from build123d import *

# Parameters (mm, degrees)
BOSS_EXTRUDE1_DEPTH = 3.5
BOSS_EXTRUDE2_DEPTH = 1.5
BOSS_EXTRUDE2_TAPER = 7


with BuildPart() as part:
    # Sketch1 → Boss-Extrude1 (new body)
    with BuildSketch(Plane.XY):
        Polygon((-2.95, 2), (-1.95, 3), (1.95, 3), (2.95, 2), (2.95, -2), (1.95, -3), (-1.95, -3), (-2.95, -2), align=None)
    extrude(amount=BOSS_EXTRUDE1_DEPTH)

    # Sketch2 → Boss-Extrude2 (add)
    with BuildSketch(Plane.XY.offset(3.5)):
        Polygon((-2.5, 1.7), (-2.5, -1.7), (-1.75, -2.45), (1.75, -2.45), (2.5, -1.7), (2.5, 1.7), (1.75, 2.45), (-1.75, 2.45), align=None)
    extrude(amount=BOSS_EXTRUDE2_DEPTH, taper=BOSS_EXTRUDE2_TAPER)


solid = part.part
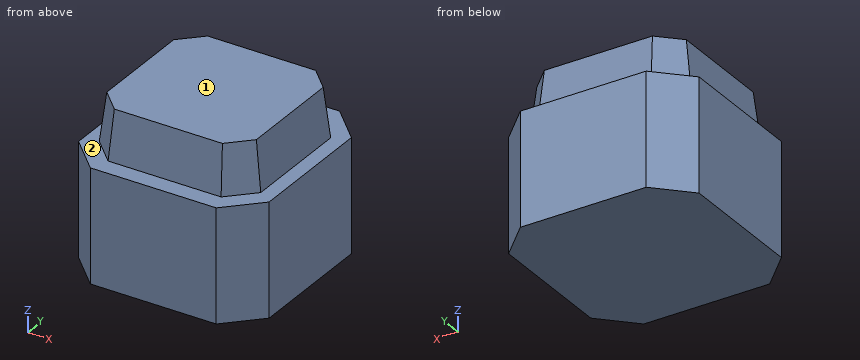
Source: CAD feature listing. Evaluate the final solid. Frame: model axes, mm. Face numbers are marked on the shaded views. A direction names the side the tool comes from. Coordinates: 2 decimals unless noted, no trailing zeros. Loops run counter-clockwise (first coordinate to the right, second up) from the corner with the lowest first, then second, coordinate; pieces in that order, holes last. Notation, with made-up numbers: (29, 83) - (61, 83) arc R9 cw to (61, 98) - close; hole circle Ø2 at (-28, 4.25). An arc over 180 degrees is marked (long way). Return JSON: item names as keys, results as strings.
Q1. Material intervals for line 1 along X through (y, z) = (-1.85, 3.7); line 2 along Z through (x, y) = (2.45, 2.4), sorted ascending.
Results:
{"line 1": "-2.32 to 2.32", "line 2": "0 to 3.5"}
Q2. Section B-B, the plane y = -0.3. Return loops of the section in (x, z).
Results:
{"outline": "(-2.95, 0) - (2.95, 0) - (2.95, 3.5) - (2.5, 3.5) - (2.32, 5) - (-2.32, 5) - (-2.5, 3.5) - (-2.95, 3.5) - close"}
Q3. Access query for the marked faces 1 and 2. Directions: +Z, -Z, +X, -X, +Y, -Y. A direction counts if a zero-diameter tool reaches every point of the face in a straight line with its end or side. Return the directions, or none.
Results:
{"face 1": "+Z, +X, -X, +Y, -Y", "face 2": "+Z"}
Q4. Section A-A, the plane x = -0.85. Return loops of the section in (y, z).
Results:
{"outline": "(-3, 0) - (3, 0) - (3, 3.5) - (2.45, 3.5) - (2.27, 5) - (-2.27, 5) - (-2.45, 3.5) - (-3, 3.5) - close"}
